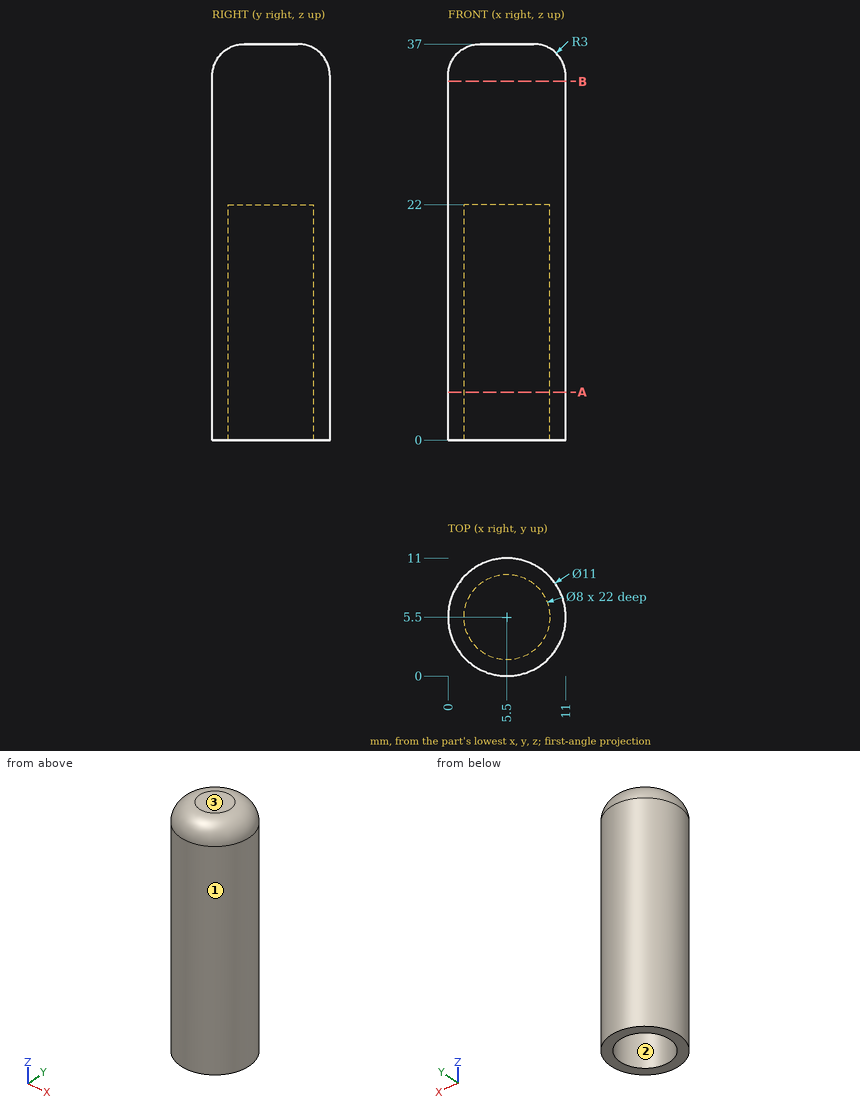
Design review of the part shown in the three views and the two pictorial views. Dimensions are in mm from the part's minimum x, y and z. Round coordinates to 2 decimals unless told otherwise and drop trailing zeros. Loops run counter-clockwise (first coordinate to the right, second up) from the corner with the lowest first, then second, coordinate; pieces in that order, holes last. Notation, with made-up numbers: (19, 20.25) -> (51, 20.25) arc R24 cw to (51, 38.25) -> close; hole circle Ø3 at (25, -37). An arc over 180 degrees is marked (long way). Answer as a JSON object with one key per item and string values. Group by question number.
1) For pin 1 Ø6 at (x, z) = (10, 30) entering from +Y; pin 2 Ø3 at (y, z) = (4, 17) entering from +X; pin 3 Ø1.5 at (x, z) = (8, 23) entering from +Y, all flat-tipped, find the tip position at first contact; note any pin that passes through.
2) For line 1 (Y direction, x = 5.5, z = 5.25); line 2 (X direction, y = 5.25, z = 17); line 3 (Y direction, x = 6.75, z = 20), list the stretches that pass through material, from the lowest coordinate up. Write a range as [from, to].
3) Mouldability with a two-part tool opening along Y and no side actions: class the marked faces 1, 2 and 3 as released by +Y, released by -Y, zero draft, split by the parting line, or undercut.
4) We need section A-A on z = 4.5. Write out the cut boundary in (x, y).
5) We need section B-B on z = 33.5. Write out the cut boundary in (x, y).
Result set:
{
 "1": {"pin 1": "y = 10.79", "pin 2": "x = 11", "pin 3": "y = 10.71"},
 "2": {"line 1": "[0, 1.5], [9.5, 11]", "line 2": "[0.01, 1.51], [9.49, 10.99]", "line 3": "[0.14, 1.7], [9.3, 10.86]"},
 "3": {"face 1": "split by the parting line", "face 2": "undercut", "face 3": "zero draft"},
 "4": {"outline": "circle Ø11 at (5.5, 5.5); hole circle Ø8 at (5.5, 5.5)"},
 "5": {"outline": "circle Ø11 at (5.5, 5.5)"}
}
